Geometry: final body of the model. Coordinates: model frame, mm. Face numbers are marked on the shaded views. Round coordinates to 2 decimals unless told otherwise and drop trailing zeros.
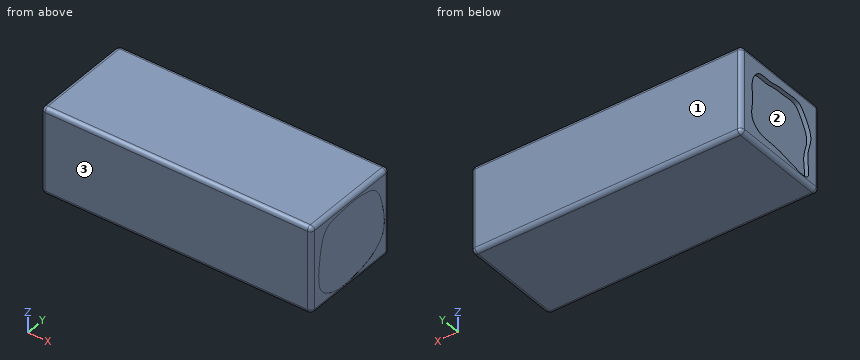
from build123d import *

# Parameters (mm, degrees)
CROQUIS2_W              = 131
CROQUIS2_H              = 42
SALIENTE_EXTRUIR1_DEPTH = 50
CORTAR_EXTRUIR1_DEPTH   = 0.02
REDONDEO1_R             = 2
CORTAR_EXTRUIR2_DEPTH   = 2


with BuildPart() as part:
    # Croquis2 → Saliente-Extruir1 (new body)
    with BuildSketch(Plane(origin=(0, 0, 0), x_dir=(1, 0, 0), z_dir=(0, 1, 0))):
        Rectangle(CROQUIS2_W, CROQUIS2_H)
    extrude(amount=SALIENTE_EXTRUIR1_DEPTH)

    # Croquis3 → Cortar-Extruir1 (cut)
    with BuildSketch(Plane(origin=(65.5, 0, 0), x_dir=(0, 0, -1), z_dir=(1, 0, 0))):
        with BuildLine():
            add(Edge.make_bspline(
                [(-17.112114557, 36.006296002), (-16.769875687, 37.42301657), (-15.057082788, 43.088866065), (-3.859638422, 46.362485269), (8.679768808, 48.154839826), (16.162022742, 38.858188467), (18.505026308, 27.939639658), (19.779716297, 16.168451708), (13.261180985, 3.841515951), (3.038463882, 4.622376827), (-6.441014061, 5.799969078), (-16.666974229, 7.476700806), (-17.543271482, 18.80297348), (-18.518864255, 27.195655921), (-17.793454872, 33.185842442), (-17.112114557, 36.006296002)],
                knots=[0, 0, 0, 0, 0.032914091, 0.131790069, 0.239123046, 0.300139284, 0.384993454, 0.497153717, 0.570211354, 0.671370628, 0.697843576, 0.799265567, 0.861163185, 0.934473554, 1, 1, 1, 1], degree=3))
        make_face()
    extrude(amount=-CORTAR_EXTRUIR1_DEPTH, mode=Mode.SUBTRACT)

    # Redondeo1
    redondeo1_edges = [part.edges().sort_by_distance(p)[0] for p in [
        (-65.5, 50, 0),
        (0, 50, 21),
        (65.5, 50, 0),
        (0, 0, 21),
        (-65.5, 0, 0),
        (0, 0, -21),
        (65.5, 0, 0),
        (0, 50, -21),
        (65.5, 25, 21),
        (-65.5, 25, 21),
        (-65.5, 25, -21),
        (65.5, 25, -21),
    ]]
    fillet(redondeo1_edges, radius=REDONDEO1_R)

    # Croquis4 → Cortar-Extruir2 (cut)
    with BuildSketch(Plane.ZY.offset(65.5)):
        with BuildLine():
            add(Edge.make_bspline(
                [(8.978661577, 42.558783476), (5.375949454, 43.867570791), (-1.149836325, 41.739656252), (-9.762030871, 44.554797073), (-16.510781784, 37.672215383), (-13.639271555, 25.861697119), (-23.105390544, 3.346347644), (-6.65065098, 8.75557637), (2.285497568, 3.421967675), (9.798682665, 8.179200373), (16.633242319, 13.22394434), (14.828389321, 19.837598078), (15.335298358, 26.153672342), (13.358929545, 31.415036468), (15.235898272, 38.524529705), (11.052519969, 41.805395623), (8.978661577, 42.558783476)],
                knots=[0, 0, 0, 0, 0.09132038, 0.159387605, 0.195313945, 0.300499967, 0.464636293, 0.542295544, 0.617262826, 0.702219659, 0.735857869, 0.814488947, 0.839285493, 0.891602027, 0.947432509, 1, 1, 1, 1], degree=3))
        make_face()
    extrude(amount=-CORTAR_EXTRUIR2_DEPTH, mode=Mode.SUBTRACT)


solid = part.part
1) First-contact query: P1, Ø3, axis at y = 34, z = -1, coming from the -X side; P2, Ø2, axis at y = 8, z = 7.5, coming from the +X side. Flat tips, straight axial feed; report the tip coordinate or a pass-through.
2) Line query: probe 1 along X at (y, z) = (21, -2.5); probe 2 along X at (y, z) = (11, 15). Output: solid intervals per line, ascending.
3) Draft query along Y for the marked faces 1, 2 and 3. Return one class per face: pulls with the +Y half, pulls with the -Y half, needs draft (parallel to the pull), parting line crosses it, or undercut.
Filled in:
1. P1: stops at x = -63.5
1. P2: stops at x = 65.48
2. probe 1: x = -63.5 to 65.48
2. probe 2: x = -65.5 to 65.48
3. face 1: pulls with the +Y half
3. face 2: undercut
3. face 3: pulls with the -Y half
